Input: part model. Units: mm. Frame: model coordinates. A direction names the side the tool comes from. Coordinates: 2 decimals unless noted, no trailing zeros. Order: outer loops, then holes, each group sorted by start corner. A loop starts at its lowest first (then second) coordinate and runs counter-clockwise, first axis right, second up. Notation, with made-up numbers: (-6, 53.25) -> (26, 53.25) arc R11 cw to (26, 64.25) -> close; hole circle Ø9 at (-6.75, 50.5). An arc over 180 degrees is marked (long way). One line per item, written item: value. Start each with the question number.
from build123d import *

# Parameters (mm, degrees)
F1_DEPTH = 60
F2_T     = -1.5


with BuildPart() as f1:
    # F0 (on Front) → F1 (new body)
    with BuildSketch(Plane.XZ):
        with BuildLine():
            Line((22.690229, 23.644435), (4.338837, 32.481999))
            ThreePointArc((4.338837, 32.481999), (0, 33.47231), (-4.338837, 32.481999))
            Line((-4.338837, 32.481999), (-22.690229, 23.644435))
            ThreePointArc((-22.690229, 23.644435), (-26.169706, 20.869644), (-28.10067, 16.859956))
            Line((-28.10067, 16.859956), (-32.63309, -2.997871))
            ThreePointArc((-32.63309, -2.997871), (-32.63309, -7.44829), (-30.702125, -11.457978))
            Line((-30.702125, -11.457978), (-18.002569, -27.382719))
            ThreePointArc((-18.002569, -27.382719), (-14.523091, -30.15751), (-10.184254, -31.147821))
            Line((-10.184254, -31.147821), (10.184254, -31.147821))
            ThreePointArc((10.184254, -31.147821), (14.523091, -30.15751), (18.002569, -27.382719))
            Line((18.002569, -27.382719), (30.702125, -11.457978))
            ThreePointArc((30.702125, -11.457978), (32.63309, -7.44829), (32.63309, -2.997871))
            Line((32.63309, -2.997871), (28.10067, 16.859956))
            ThreePointArc((28.10067, 16.859956), (26.169706, 20.869644), (22.690229, 23.644435))
        make_face()
    extrude(amount=F1_DEPTH)

    # F2
    f2_openings = [f1.faces().sort_by_distance(p)[0] for p in [
        (0, -60, 0),
    ]]
    offset(amount=F2_T, openings=f2_openings)


solid = f1.part
1) Ray query, line 1 along X through (y, z) = (-4.5, -10.5); line 2 along Y through (x, z) = (-7, -18); line 3 along X through (y, z) = (-20.5, 13). Return the intervals inside material, ascending. Write a range as from..to.
2) Section query B-B, the plane z = -5.5. Return the cut outline in (x, y).
3) Pin query (flat end, axial travel): pin 1 Ø2 at (y, z) = (-29.5, 9) entering from +X; pin 2 Ø5 at (x, y) = (14.5, -15) entering from +Z; pin 3 Ø4 at (x, y) = (15, -37.5) entering from +Z; pin 4 Ø10 at (y, z) = (-10.5, -1) entering from +X. Return the tip coordinate at first contact, or that it passes through.
4) Access query for faces 1 (the cylindrical face through (31.159, -30.34, -7.167)), 2 (the flat face through (0, -60, -30)). Directions: +Z, -Z, +X, -X, +Y, -Y. A direction counts if a zero-diameter tool reaches every point of the face in a straight line with its end or side. Return the directions, or none.
5) Section query C-C, the plane x = 24. Return the cut outline in (y, z), plus the area to 3 significant figures.
6) Mould query, pull axis Z, two halves, no side actions, for faces 3 (the cylindrical face through (-26.13, -29.58, 20.92)), 4 (the flat face through (28.936, -30.34, 6.458)), 5 (the flat face through (-24.44, -29.58, -19.31)). Classes: +Z half, -Z half, draft (parallel to the pull), parting line (faces both ways), or undercut.
7) Section query A-A, the plane y = -44. Return the cut outline in (x, z), plus the area to 3 significant figures.
Entries:
1. line 1: x = -31.38..-29.55, 29.55..31.38
1. line 2: y = -1.5..0
1. line 3: x = -28.98..-27.44, 27.44..28.98
2. outline: (-32.88, -60) -> (-31.38, -60) -> (-31.38, -1.5) -> (31.38, -1.5) -> (31.38, -60) -> (32.88, -60) -> (32.88, 0) -> (-32.88, 0) -> close
3. pin 1: stops at x = 30.12
3. pin 2: stops at z = 28.79
3. pin 3: stops at z = 28.31
3. pin 4: stops at x = 32.88
4. face 1: -Y
4. face 2: +Z, -Z, +X, -X, -Y
5. outline: (-60, -19.86) -> (0, -19.86) -> (0, 22.89) -> (-60, 22.89) -> (-60, 20.99) -> (-1.5, 20.99) -> (-1.5, -17.46) -> (-60, -17.46) -> close
5. area: 316 mm2
6. face 3: +Z half
6. face 4: undercut
6. face 5: -Z half
7. outline: (-32.63, -3) arc R10 ccw to (-30.7, -11.46) -> (-18, -27.38) arc R10 ccw to (-10.18, -31.15) -> (10.18, -31.15) arc R10 ccw to (18, -27.38) -> (30.7, -11.46) arc R10 ccw to (32.63, -3) -> (28.1, 16.86) arc R10 ccw to (22.69, 23.64) -> (4.34, 32.48) arc R10 ccw to (-4.34, 32.48) -> (-22.69, 23.64) arc R10 ccw to (-28.1, 16.86) -> close; hole (-31.17, -3.33) arc R8.5 ccw to (-29.53, -10.52) -> (-16.83, -26.45) arc R8.5 ccw to (-10.18, -29.65) -> (10.18, -29.65) arc R8.5 ccw to (16.83, -26.45) -> (29.53, -10.52) arc R8.5 ccw to (31.17, -3.33) -> (26.64, 16.53) arc R8.5 ccw to (22.04, 22.29) -> (3.69, 31.13) arc R8.5 ccw to (-3.69, 31.13) -> (-22.04, 22.29) arc R8.5 ccw to (-26.64, 16.53) -> close
7. area: 301 mm2
